Geometry: final body of the model. Coordinates: model frame, mm. Give positions to 0.01 mm unless a question says otherwise; leave off trailing zeros. Loops run counter-clockwise (first coordinate to the right, second up) from the corner with the lowest first, then second, coordinate; pieces in that order, holes last.
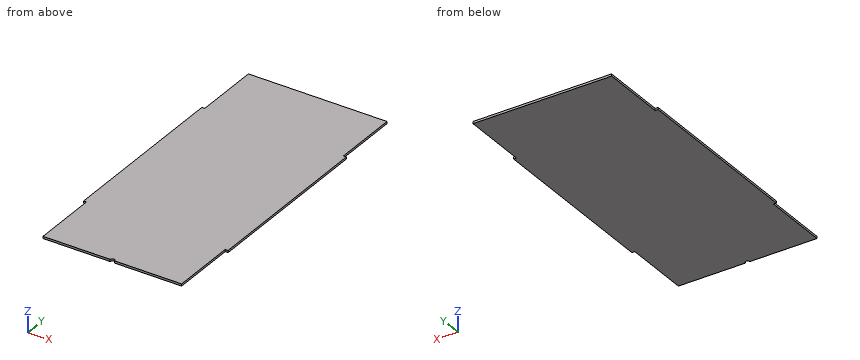
Autodesk Inventor part; units mm, degrees
ref_plane "YZ Plane" through (0, 0, 0) normal (1, 0, 0) x (0, 1, 0)
ref_plane "XZ Plane" through (0, 0, 0) normal (0, 1, 0) x (-1, 0, 0)
ref_plane "XY Plane" through (0, 0, 0) normal (0, 0, 1) x (1, 0, 0)
sketch "Sketch1" plane through (0, 0, 0) normal (0, 0, 1) x (1, 0, 0)
  line L0 (-96.5, -217) -> (96.5, -217)
  line L1 (96.5, -217) -> (96.5, 217)
  line L2 (-96.5, 217) -> (-96.5, -217)
  line L3 (-96.5, -217) -> (96.5, 217) construction
  line L4 (96.5, -217) -> (-96.5, 217) construction
  line L5 (-96.5, 217) -> (96.5, 217)
  line L6 (-96.5, 125) -> (-100.5, 125)
  line L7 (-100.5, 125) -> (-100.5, -125)
  line L8 (-100.5, -125) -> (-96.5, -125)
  line L9 (-96.5, -125) -> (-96.5, 125)
  line L10 (0, 217) -> (0, 0)
  line L11 (96.5, 125) -> (100.5, 125)
  line L12 (100.5, 125) -> (100.5, -125)
  line L13 (100.5, -125) -> (96.5, -125)
  line L14 (96.5, -125) -> (96.5, 125)
  point P0 (-100.5, 0)
  point P1 (-96.5, 0)
  point P2 (-96.5, -125)
  point P3 (100.5, 0)
  point P4 (96.5, 0)
  point P5 (96.5, 125)
  point P6 (96.5, -125)
  dimension "d0" = 434
  dimension "d1" = 193
  dimension "d3" = 4
  dimension "d4" = 250
extrude "Plate1" add sketch "Sketch1" along normal blind 3
sketch "Sketch2" plane through (0, 0, 3) normal (0, 0, 1) x (1, 0, 0)
  line L0 (-96.5, -217) -> (96.5, -217)
  arc A0 (3, -217) -> (-3, -217) centre (0, -217) ccw
  line L1 (96.5, -217) -> (-96.5, -217)
  point P0 (0, 0)
  dimension "d6" = 3
extrude "Cut1" cut sketch "Sketch2" against normal blind 3
equation "\"d7\" = Thickness"
equation "\"d5\" = Thickness"
equation "\"BendRadius\" = Thickness"
equation "\"BendReliefWidth\" = Thickness"
equation "\"BendReliefDepth\" = 0.5 * Thickness"
equation "\"CornerReliefSize\" = 4 * Thickness"
equation "\"MinimumRemnant\" = 2 * Thickness"
equation "\"TransitionRadius\" = BendRadius"
equation "\"JacobiRadiusSize\" = BendRadius"
equation "\"GapSize\" = Thickness"
properties part number "Finishing Sheets .3  ( Back )"
Item 1: Ray query, probe 1 along X at (y, z) = (-164, 0.95); probe 2 along Y at (x, z) = (2.5, 1.55). Return the intervals inside material, ascending.
Values follow:
probe 1: x = -96.5 to 96.5
probe 2: y = -215.34 to 217
Item 2: Pin query (flat end, axial travel): pin 1 (1.5 mm diameter, centred on x = -98, z = 1.5, fed in from +Y); pin 2 (0.9 mm diameter, centred on y = 177.5, z = 1, fed in from -X); pin 3 (8 mm diameter, centred on x = 71, y = -101.5, fed in from -Z); pin 4 (0.9 mm diameter, centred on x = 97.5, z = 2, fed in from -Y). Return the tip coordinate at first contact, or that it passes through.
Values follow:
pin 1: stops at y = 125
pin 2: stops at x = -96.5
pin 3: stops at z = 0
pin 4: stops at y = -125
Item 3: Section query A-A on z = 1.2. Return loops of the section in (x, y).
Values follow:
outline: (-100.5, -125) - (-96.5, -125) - (-96.5, -217) - (-3, -217) arc R3 cw to (3, -217) - (96.5, -217) - (96.5, -125) - (100.5, -125) - (100.5, 125) - (96.5, 125) - (96.5, 217) - (-96.5, 217) - (-96.5, 125) - (-100.5, 125) - close
Item 4: Section query B-B on y = 146.5. Return loops of the section in (x, z), plus the area to 3 significant figures.
Values follow:
outline: (-96.5, 0) - (96.5, 0) - (96.5, 3) - (-96.5, 3) - close
area: 579 mm2
